```python
from build123d import *

# Parameters (mm, degrees)
SKETCH1_R                  = 4
BOSS_EXTRUDE1_DEPTH        = 9.525
FILLET1_R                  = 10
M8X1_25_TAPPED_HOLE1_D     = 6.8
M8X1_25_TAPPED_HOLE1_DEPTH = 32.25
M8X1_25_TAPPED_HOLE1_TIP   = 2.042926105
FILLET2_R                  = 2


with BuildPart() as part:
    # Sketch1 → Boss-Extrude1 (new body)
    with BuildSketch(Plane(origin=(0, 0, 0), x_dir=(1, 0, 0), z_dir=(0, 1, 0))):
        with BuildLine():
            Line((-7, 40), (7, 40))
            Line((7, 40), (7, 3.872983346))
            ThreePointArc((7, 3.872983346), (8, 0), (7, -3.872983346))
            Line((7, -3.872983346), (7, -13.872983346))
            Line((7, -13.872983346), (37.5, -35))
            Line((37.5, -35), (37.5, -40))
            ThreePointArc((37.5, -40), (26.579328871, -47.956118241), (14.044571905, -53))
            Line((14.044571905, -53), (-14.044571905, -53))
            ThreePointArc((-14.044571905, -53), (-26.579328871, -47.956118241), (-37.5, -40))
            Line((-37.5, -40), (-37.5, -35))
            Line((-37.5, -35), (-7, -13.872983346))
            Line((-7, -13.872983346), (-7, -3.872983346))
            ThreePointArc((-7, -3.872983346), (-8, 0), (-7, 3.872983346))
            Line((-7, 3.872983346), (-7, 40))
        make_face()
        Circle(SKETCH1_R, mode=Mode.SUBTRACT)
    extrude(amount=BOSS_EXTRUDE1_DEPTH)

    # Fillet1
    fillet1_edges = [part.edges().sort_by_distance(p)[0] for p in [
        (7, 4.7625, -3.872983346),
        (7, 4.7625, 3.872983346),
        (-7, 4.7625, 3.872983346),
        (-7, 4.7625, -3.872983346),
    ]]
    fillet(fillet1_edges, radius=FILLET1_R)

    # M8x1.25 Tapped Hole1
    with Locations(Plane(origin=(0, 0, -40), x_dir=(-1, 0, 0), z_dir=(0, 0, -1))):
        with Locations((0, 4.7625)):
            Hole(M8X1_25_TAPPED_HOLE1_D / 2, depth=M8X1_25_TAPPED_HOLE1_DEPTH)
            with Locations((0, 0, -(M8X1_25_TAPPED_HOLE1_DEPTH + M8X1_25_TAPPED_HOLE1_TIP / 2))):  # 118° drill point
                Cone(0, M8X1_25_TAPPED_HOLE1_D / 2, M8X1_25_TAPPED_HOLE1_TIP, mode=Mode.SUBTRACT)

    # Fillet2
    fillet2_edges = [part.edges().sort_by_distance(p)[0] for p in [
        (7, 4.7625, 13.872983346),
        (37.5, 4.7625, 35),
        (37.5, 4.7625, 40),
        (-37.5, 4.7625, 40),
        (-37.5, 4.7625, 35),
        (-7, 4.7625, 13.872983346),
    ]]
    fillet(fillet2_edges, radius=FILLET2_R)


solid = part.part
```
Verification items for the finished model (mm, model axes). A direction names the side the tool comes from. Round coordinates to 2 decimals unless told otherwise and drop trailing zeros. Order: outer loops, then holes, each group sorted by start corner. A loop starts at its lowest first (then second) coordinate and runs counter-clockwise, first axis right, second up. Notation, with made-up numbers: (-9, 1) -> (28, 1) arc R18 ccw to (28, 25) -> close; hole circle Ø7 at (16.25, 31.25). An arc over 180 degrees is marked (long way). Put each result on its own line as item: value. Start each with the question number.
(1) Section check C-C (x = 16.5). Enter the section's corners in (y, z) (3 decimals).
(2) Section check B-B (z = 9.5). Enter the section's corners in (x, y) (3 decimals).
(3) Material ranges on line 1 along X through (y, z) = (6.75, 0); line 2 along Z through (x, y) = (3, 6.75); line 3 along Y through (x, z) = (0, -31) (1 decimal), recorded low to high.
(4) Tool access check on faces 1 (the face through (-1.7, 1.5, -40)), 2 (the face through (-26.027, 4.696, 48.258)), 3 (the face through (-7, 5, 9)), 4 (the face through (7.144, 4.829, 4.226)), 5 (the face through (-7, 5, -23)). Record the directions out of +Z, -Z, +X, -X, +Y, -Y that give a thin tool (end or side, any length) a straight path to the whole face; none if there is none.
(5) Draft check along Z on faces 6 (the face through (-0.443, 8.134, -23.649)), 7 (the face through (7, 5, 9)), 8 (the face through (7.136, 4.829, -4.273)). Enter one of: +Z half, -Z half, draft (parallel to the pull), parting line (faces both ways), or undercut.
(6) Depth check by flat-ended pin: pin 1 Ø2 at (x, y) = (-15.5, 1.5) entering from -Z; pin 2 Ø1 at (x, z) = (12.5, 15) entering from +Y; pin 3 Ø3 at (y, z) = (4, -28) entering from -X; pin 4 Ø1.5 at (y, z) = (2, 2.5) entering from -X. Enter the tip coordinate at first touch or a pass-through.
(7) Section check A-A (z = 0). Enter the section's corners in (x, y) (3 decimals), then the cut area to 3 significant figures.
Completed:
1. outline: (0, 20.454) -> (9.525, 20.454) -> (9.525, 52.288) -> (0, 52.288) -> close
2. outline: (-7, 0) -> (7, 0) -> (7, 9.525) -> (-7, 9.525) -> close
3. line 1: x = -8 to -4, 4 to 8
3. line 2: z = -40 to -2.65, 2.65 to 53
3. line 3: y = 0 to 1.4, 8.2 to 9.5
4. face 1: -Z, +X, -X, +Y, -Y
4. face 2: +Z, -X, +Y, -Y
4. face 3: -X, +Y, -Y
4. face 4: +X, +Y, -Y
4. face 5: -Z, -X, +Y, -Y
5. face 6: draft
5. face 7: undercut
5. face 8: -Z half
6. pin 1: stops at z = 19.07
6. pin 2: passes through
6. pin 3: stops at x = -7
6. pin 4: stops at x = -7.81
7. outline: (-8, 0) -> (-4, 0) -> (-4, 9.525) -> (-8, 9.525) -> close; (4, 0) -> (8, 0) -> (8, 9.525) -> (4, 9.525) -> close
7. area: 76.2 mm2
